Here's how the part is built. I have some questions about the finished solid (model axes, mm). Coordinates: 2 decimals unless noted, no trailing zeros. Write each loop counter-clockwise with the first axis right and the second up, starting at its lowest first coordinate (ties: lowest second). Pieces come first, ordered by that corner, then holes.
(1) Imagine slicing it at A-A, the plane z = 39. List the corners of the cut face in (x, y) for me, plus the area to 3 significant figures.
(2) For pin 1 Ø1.5 at (x, z) = (-443.5, 76) entering from -Y; pin 2 Ø18 at (y, z) = (-63.5, 113) entering from +X; pin 3 Ø18 at (x, z) = (-14.5, 107.5) entering from -Y, each with a flat end and sliding along its axis, tell me the tip position at first contact or that it passes through.
(3) Please list where these lines run through material, in increasing order: probe 1 along X at (y, z) = (-292.5, 88.5); probe 2 along Y at (x, z) = (-295, 37); probe 3 along X at (y, z) = (-113, 17.5).
(4) Imagine slicing it at B-B, the plane y = 103.5. List the corners of the cut face in (x, z) for me.
(5) Imagine slicing it at C-C, the plane x = -139. State how many separate pieces and enclosed holes the cut face has, plus the area to 3 significant figures.
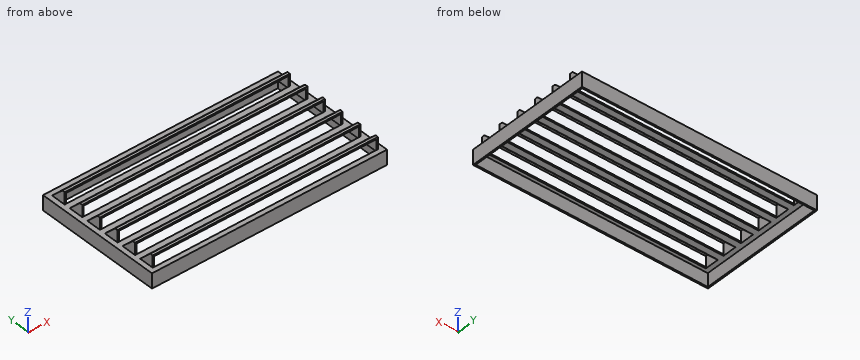
```python
from build123d import *

# Parameters (mm, degrees)
F0_W         = 1200
F0_H         = 650
F1_DEPTH     = 75
F3_START     = -25
F3_DEPTH     = 1150
F4_T         = 7.5
F4_T3_DEPTH  = 90
F4_T5_DEPTH  = 1165
F4_T7_DEPTH  = 90
F4_T9_DEPTH  = 90
F4_T11_DEPTH = 90
F4_T13_DEPTH = 90
F4_T15_DEPTH = 90


# Not quite as in the source:
# - a shell that OpenCascade refuses in one call is made with other operations: the cavity is built on its own and cut out
# - a feature names something its author has since deleted; it is built from what else it names


with BuildPart() as f1:
    # F0 (on Top) → F1 (new body)
    with BuildSketch(Plane.XY):
        Rectangle(F0_W, F0_H)
    extrude(amount=F1_DEPTH)

    # F2 (on face) → F3 (join)
    with BuildSketch(Plane(origin=(-600, 0, 0), x_dir=(0, -1, 0), z_dir=(-1, 0, 0)).offset(F3_START)):
        Polygon((-239.4699645042, 135.5300354958), (-300, 75), (-225, 75), (-225, 135.5300354958), align=None)
        Polygon((-134.4699645042, 135.5300354958), (-195, 75), (-120, 75), (-120, 135.5300354958), align=None)
        Polygon((-29.4699645042, 135.5300354958), (-90, 75), (-15, 75), (-15, 135.5300354958), align=None)
        Polygon((75.5300354958, 135.5300354958), (15, 75), (90, 75), (90, 135.5300354958), align=None)
        Polygon((120, 75), (195, 75), (195, 135.5300354958), (180.5300354958, 135.5300354958), align=None)
        Polygon((225, 75), (300, 75), (300, 135.5300354958), (285.5300354958, 135.5300354958), align=None)
    extrude(amount=-F3_DEPTH)

    # F4: shell of thickness 7.5, made by hand


with BuildPart() as f4_core1:
    # F4_t2: copy of F1
    add(f1.part)

    # the walls: a layer under each face that stays
    f4_faces = [f4_core1.faces().sort_by_distance(p)[0] for p in [
        (0, -325, 37.5),
        (-600, 0, 37.5),
        (600, 0, 37.5),
        (0, 0, 75),
        (0, 325, 37.5),
        (-575, -262.5, 105.2650177479),
        (575, -262.5, 105.2650177479),
        (0, -255.2650177479, 105.2650177479),
        (-575, -157.5, 105.2650177479),
        (575, -157.5, 105.2650177479),
        (0, -150.2650177479, 105.2650177479),
        (-575, -52.5, 105.2650177479),
        (575, -52.5, 105.2650177479),
        (0, -45.2650177479, 105.2650177479),
        (-575, 52.5, 105.2650177479),
        (575, 52.5, 105.2650177479),
        (0, 59.7349822521, 105.2650177479),
        (-575, 157.5, 105.2650177479),
        (575, 157.5, 105.2650177479),
        (0, 164.7349822521, 105.2650177479),
        (-575, 262.5, 105.2650177479),
        (575, 262.5, 105.2650177479),
        (0, 269.7349822521, 105.2650177479),
        (0, -292.7650177479, 135.5300354958),
        (0, -187.7650177479, 135.5300354958),
        (0, -82.7650177479, 135.5300354958),
        (0, 22.2349822521, 135.5300354958),
        (0, 127.2349822521, 135.5300354958),
        (0, 232.2349822521, 135.5300354958),
    ]]
    thicken(f4_faces, amount=-F4_T, mode=Mode.SUBTRACT)

    # F4_s4 → F4_t3 (cut)
    with BuildSketch(Plane.XZ.offset(217.5)):
        Polygon((-575.075, 75.075), (-575, 67.5), (-567.5, 67.5), (-567.5, 75), align=None)
        Polygon((575.075, 75.075), (575, 67.5), (567.5, 67.5), (567.5, 75), align=None)
    extrude(amount=F4_T3_DEPTH, mode=Mode.SUBTRACT)

    # F4_s6 → F4_t5 (cut)
    with BuildSketch(Plane.YZ.offset(-582.5)):
        Polygon((-224.9469669914, 75.1280330086), (-225, 67.5), (-228.1066017178, 67.5), (-230.3033008589, 69.6966991411), align=None)
        Polygon((-119.9469669914, 75.1280330086), (-120, 67.5), (-123.1066017178, 67.5), (-125.3033008589, 69.6966991411), align=None)
        Polygon((-14.9469669914, 75.1280330086), (-15, 67.5), (-18.1066017178, 67.5), (-20.3033008589, 69.6966991411), align=None)
        Polygon((90.0530330086, 75.1280330086), (90, 67.5), (86.8933982822, 67.5), (84.6966991411, 69.6966991411), align=None)
        Polygon((195.0530330086, 75.1280330086), (195, 67.5), (191.8933982822, 67.5), (189.6966991411, 69.6966991411), align=None)
        Polygon((300.0530330086, 75.1280330086), (300, 67.5), (296.8933982822, 67.5), (294.6966991411, 69.6966991411), align=None)
    extrude(amount=F4_T5_DEPTH, mode=Mode.SUBTRACT)

    # F4_s8 → F4_t7 (cut)
    with BuildSketch(Plane.XZ.offset(112.5)):
        Polygon((-575.075, 75.075), (-575, 67.5), (-567.5, 67.5), (-567.5, 75), align=None)
        Polygon((575.075, 75.075), (575, 67.5), (567.5, 67.5), (567.5, 75), align=None)
    extrude(amount=F4_T7_DEPTH, mode=Mode.SUBTRACT)

    # F4_s10 → F4_t9 (cut)
    with BuildSketch(Plane.XZ.offset(7.5)):
        Polygon((-575.075, 75.075), (-575, 67.5), (-567.5, 67.5), (-567.5, 75), align=None)
        Polygon((575.075, 75.075), (575, 67.5), (567.5, 67.5), (567.5, 75), align=None)
    extrude(amount=F4_T9_DEPTH, mode=Mode.SUBTRACT)

    # F4_s12 → F4_t11 (cut)
    with BuildSketch(Plane.XZ.offset(-97.5)):
        Polygon((-575.075, 75.075), (-575, 67.5), (-567.5, 67.5), (-567.5, 75), align=None)
        Polygon((575.075, 75.075), (575, 67.5), (567.5, 67.5), (567.5, 75), align=None)
    extrude(amount=F4_T11_DEPTH, mode=Mode.SUBTRACT)

    # F4_s14 → F4_t13 (cut)
    with BuildSketch(Plane.XZ.offset(-202.5)):
        Polygon((-575.075, 75.075), (-575, 67.5), (-567.5, 67.5), (-567.5, 75), align=None)
        Polygon((575.075, 75.075), (575, 67.5), (567.5, 67.5), (567.5, 75), align=None)
    extrude(amount=F4_T13_DEPTH, mode=Mode.SUBTRACT)

    # F4_s16 → F4_t15 (cut)
    with BuildSketch(Plane.XZ.offset(-307.5)):
        Polygon((-575.075, 75.075), (-575, 67.5), (-567.5, 67.5), (-567.5, 75), align=None)
        Polygon((575.075, 75.075), (575, 67.5), (567.5, 67.5), (567.5, 75), align=None)
    extrude(amount=F4_T15_DEPTH, mode=Mode.SUBTRACT)


with BuildPart() as f1_1:
    add(f1.part)

    # what is left inside the walls is the cavity
    f4_cavity = [f4_core1.part.solids().sort_by_distance(p)[0] for p in [
        (0, -105.833333, 0.075),
    ]]
    add(f4_cavity, mode=Mode.SUBTRACT)


solid = f1_1.part
```
Recorded:
1. outline: (-600, -325) - (600, -325) - (600, 325) - (-600, 325) - close; hole (-592.5, -317.5) - (592.5, -317.5) - (592.5, 317.5) - (-592.5, 317.5) - close
1. area: 27,500 mm2
2. pin 1: stops at y = -237.36
2. pin 2: stops at x = 575
2. pin 3: stops at y = -277.11
3. probe 1: x = -575 to -567.5, 567.5 to 575
3. probe 2: y = -325 to -317.5, 317.5 to 325
3. probe 3: x = -600 to -592.5, 592.5 to 600
4. outline: (-600, 0) - (-592.5, 0) - (-592.5, 67.5) - (592.5, 67.5) - (592.5, 0) - (600, 0) - (600, 75) - (-600, 75) - close
5. separate pieces: 7
5. enclosed holes: 0
5. area: 7,020 mm2
